Here's how the part is built. I have some questions about the finished solid (model axes, mm). A direction names the side the tool comes from. Round coordinates to 2 decimals unless told otherwise and drop trailing zeros. Loops run counter-clockwise (first coordinate to the right, second up) from the corner with the lowest first, then second, coordinate; pieces in that order, holes last. Notation, with made-up numbers: (8, 44) - (34, 44) arc R30 ccw to (34, 74) - close; hole circle Ø8 at (-24.75, -0.75). An arc over 180 degrees is marked (long way). Return JSON: item names as keys, results as strings. Group by question number.
```python
from build123d import *

# Parameters (mm, degrees)
SKETCH001_W  = 6
SKETCH001_H  = 6
PAD001_DEPTH = 0.1
FILLET001_R  = 0.3
PAD008_DEPTH = 0.7
FILLET003_R  = 0.29
PAD009_DEPTH = 0.7
FILLET004_R  = 0.29
PAD010_DEPTH = 0.7
FILLET005_R  = 0.29
SKETCH_W     = 6
SKETCH_H     = 6
PAD_DEPTH    = 3.5
FILLET_R     = 0.3
SKETCH004_R  = 0.5
PAD003_DEPTH = 0.6
SKETCH003_R  = 0.5
PAD004_DEPTH = 0.6
SKETCH005_R  = 0.5
PAD002_DEPTH = 0.6
SKETCH002_R  = 0.5
PAD005_DEPTH = 0.6
SKETCH006_R  = 1.75
PAD006_DEPTH = 0.8
FILLET006_R  = 0.1
PAD007_DEPTH = 0.7
FILLET002_R  = 0.29


with BuildPart() as fillet001:
    # Sketch001 → Pad001 (new body)
    with BuildSketch(Plane.XY.offset(3.5)):
        with Locations((3.15, -2.25)):
            Rectangle(SKETCH001_W, SKETCH001_H)
    extrude(amount=PAD001_DEPTH)

    # Fillet001
    fillet001_edges = [fillet001.edges().sort_by_distance(p)[0] for p in [
        (6.15, -5.25, 3.55),
        (0.15, -5.25, 3.55),
        (6.15, 0.75, 3.55),
        (0.15, 0.75, 3.55),
    ]]
    fillet(fillet001_edges, radius=FILLET001_R)


with BuildPart() as fillet003:
    # Sketch008 → Pad008 (new body)
    with BuildSketch(Plane.XZ.offset(0.35)):
        Polygon((-0.15, 1.5), (0.15, 1.5), (0.15, -0.5), (-0.15, -1.5), (0.15, -2.5), (0.15, -3.5), (-0.15, -3.5), (-0.15, -2.5), (-0.45, -1.5), (-0.15, -0.5), align=None)
    extrude(amount=-PAD008_DEPTH)

    # Fillet003
    fillet003_edges = [fillet003.edges().sort_by_distance(p)[0] for p in [
        (-0.15, 0, -2.5),
        (-0.15, 0, -0.5),
        (-0.45, 0, -1.5),
        (-0.15, 0, 1.5),
        (0.15, 0, -0.5),
        (-0.15, 0, -1.5),
        (0.15, 0, -2.5),
    ]]
    fillet(fillet003_edges, radius=FILLET003_R)


with BuildPart() as fillet004:
    # Sketch009 → Pad009 (new body)
    with BuildSketch(Plane.XZ.offset(4.85)):
        Polygon((6.45, 1.5), (6.15, 1.5), (6.15, -0.5), (6.45, -1.5), (6.15, -2.5), (6.15, -3.5), (6.45, -3.5), (6.45, -2.5), (6.75, -1.5), (6.45, -0.5), align=None)
    extrude(amount=-PAD009_DEPTH)

    # Fillet004
    fillet004_edges = [fillet004.edges().sort_by_distance(p)[0] for p in [
        (6.45, -4.5, -2.5),
        (6.45, -4.5, -0.5),
        (6.75, -4.5, -1.5),
        (6.45, -4.5, 1.5),
        (6.15, -4.5, -0.5),
        (6.45, -4.5, -1.5),
        (6.15, -4.5, -2.5),
    ]]
    fillet(fillet004_edges, radius=FILLET004_R)


with BuildPart() as fillet005:
    # Sketch010 → Pad010 (new body)
    with BuildSketch(Plane.XZ.offset(0.35)):
        Polygon((6.45, 1.5), (6.15, 1.5), (6.15, -0.5), (6.45, -1.5), (6.15, -2.5), (6.15, -3.5), (6.45, -3.5), (6.45, -2.5), (6.75, -1.5), (6.45, -0.5), align=None)
    extrude(amount=-PAD010_DEPTH)

    # Fillet005
    fillet005_edges = [fillet005.edges().sort_by_distance(p)[0] for p in [
        (6.45, 0, -2.5),
        (6.45, 0, -0.5),
        (6.75, 0, -1.5),
        (6.45, 0, 1.5),
        (6.15, 0, -0.5),
        (6.45, 0, -1.5),
        (6.15, 0, -2.5),
    ]]
    fillet(fillet005_edges, radius=FILLET005_R)


with BuildPart() as fillet_body:
    # Sketch → Pad (new body)
    with BuildSketch(Plane.XY):
        with Locations((3.15, -2.25)):
            Rectangle(SKETCH_W, SKETCH_H)
    extrude(amount=PAD_DEPTH)

    # Fillet
    fillet_edges = [fillet_body.edges().sort_by_distance(p)[0] for p in [
        (6.15, 0.75, 1.75),
        (6.15, -5.25, 1.75),
        (0.15, -5.25, 1.75),
        (0.15, 0.75, 1.75),
    ]]
    fillet(fillet_edges, radius=FILLET_R)


with BuildPart() as pad003:
    # Pad003 base: copy of Fillet body
    add(fillet_body.part)

    # Sketch004 → Pad003 (new body)
    with BuildSketch(Plane.XY.offset(3.5)):
        with Locations((5.15, -0.25)):
            Circle(SKETCH004_R)
    extrude(amount=PAD003_DEPTH)


with BuildPart() as pad004:
    # Pad004 base: copy of Fillet body
    add(fillet_body.part)

    # Sketch003 → Pad004 (new body)
    with BuildSketch(Plane.XY.offset(3.5)):
        with Locations((5.15, -4.25)):
            Circle(SKETCH003_R)
    extrude(amount=PAD004_DEPTH)


with BuildPart() as pad002:
    # Pad002 base: copy of Fillet body
    add(fillet_body.part)

    # Sketch005 → Pad002 (new body)
    with BuildSketch(Plane.XY.offset(3.5)):
        with Locations((1.15, -0.25)):
            Circle(SKETCH005_R)
    extrude(amount=PAD002_DEPTH)


with BuildPart() as pad005:
    # Pad005 base: copy of Fillet body
    add(fillet_body.part)

    # Sketch002 → Pad005 (new body)
    with BuildSketch(Plane.XY.offset(3.5)):
        with Locations((1.15, -4.25)):
            Circle(SKETCH002_R)
    extrude(amount=PAD005_DEPTH)


with BuildPart() as fillet006:
    # Pad006 base: copy of Fillet body
    add(fillet_body.part)

    # Sketch006 → Pad006 (new body)
    with BuildSketch(Plane.XY.offset(3.5)):
        with Locations((3.15, -2.25)):
            Circle(SKETCH006_R)
    extrude(amount=PAD006_DEPTH)

    # Fillet006
    fillet006_edges = [fillet006.edges().sort_by_distance(p)[0] for p in [
        (1.4, -2.25, 4.3),
    ]]
    fillet(fillet006_edges, radius=FILLET006_R)


with BuildPart() as obj1:
    # Sketch007 → Pad007 (new body)
    with BuildSketch(Plane.XZ.offset(4.85)):
        Polygon((-0.15, 1.5), (0.15, 1.5), (0.15, -0.5), (-0.15, -1.5), (0.15, -2.5), (0.15, -3.5), (-0.15, -3.5), (-0.15, -2.5), (-0.45, -1.5), (-0.15, -0.5), align=None)
    extrude(amount=-PAD007_DEPTH)

    # Fillet002
    fillet002_edges = [obj1.edges().sort_by_distance(p)[0] for p in [
        (-0.15, -4.5, -2.5),
        (-0.15, -4.5, -0.5),
        (-0.45, -4.5, -1.5),
        (-0.15, -4.5, 1.5),
        (0.15, -4.5, -0.5),
        (-0.15, -4.5, -1.5),
        (0.15, -4.5, -2.5),
    ]]
    fillet(fillet002_edges, radius=FILLET002_R)

    add(fillet001.part)
    add(fillet003.part)
    add(fillet004.part)
    add(fillet005.part)
    add(pad003.part)
    add(pad004.part)
    add(pad002.part)
    add(pad005.part)
    add(fillet006.part)


solid = obj1.part
```
Q1. Imagine slicing it at D-D, the plane z = -1.75. List the corners of the cut face in (x, y) for me (3 decimals), and give its area (3 significant figures).
Q2. Imagine slicing it at A-A, the plane z = 1. List the corners of the cut face in (x, y) for me.
Q3. For faces 4 (the flat face through (3, -2, 0)), 5 (the flat face through (5, -4, 4.1)), 6 (the flat face through (6.15, -2, 2)), 7 (the cylindrical face through (5.627, -0.1, 3.846)), 8 (the flat face through (0.15, -2, 2)), which set-ups out of +Z, -Z, +X, -X, +Y, -Y let a thin tool reach every point of the face, with its end or its side?
Q4. If we mould it in two halves opening along Y, with no side actions, what happens to faces 1 (the cylindrical face through (1.627, -0.1, 3.846)), 2 (the flat face through (3, -5.25, 2)), 3 (the flat face through (1, -4, 4.1))? For each: +Y half, -Y half, draft (parallel to the pull), parting line (faces both ways), or undercut.
Q5. Imagine slicing it at C-C, the plane x = 3.15. List the corners of the cut face in (y, z) for me.
Q6. Imagine slicing it at B-B, the plane y = -2.25. List the corners of the cut face in (x, z) for me, and give its area (3 significant figures).
Q7. Please list where these lines run through material, in increasing order: line 1 (X direction, y = -0.2, z = -2.75); line 2 (Z direction, x = 4, y = -2.55); line 3 (X direction, y = -3.3, z = 1).
Q8. Will these pins go through, and if not, where does the flat tip stop? pin 1 Ø0.6 at (y, z) = (-4.5, -3) entering from -X; pin 2 Ø0.6 at (y, z) = (0, 0.5) entering from +X; pin 3 Ø1.8 at (y, z) = (-1, 1.5) entering from -X; pin 4 Ø1 at (x, y) = (5, -1.5) entering from +Z.
Output values:
{
 "1": {"outline": "(-0.375, -4.85) - (-0.075, -4.85) - (-0.075, -4.15) - (-0.375, -4.15) - close; (-0.375, -0.35) - (-0.075, -0.35) - (-0.075, 0.35) - (-0.375, 0.35) - close; (6.375, -4.85) - (6.675, -4.85) - (6.675, -4.15) - (6.375, -4.15) - close; (6.375, -0.35) - (6.675, -0.35) - (6.675, 0.35) - (6.375, 0.35) - close", "area": "0.840 mm^2"},
 "2": {"outline": "(-0.15, -4.85) - (0.15, -4.85) - (0.15, -4.95) arc R0.3 ccw to (0.45, -5.25) - (5.85, -5.25) arc R0.3 ccw to (6.15, -4.95) - (6.15, -4.85) - (6.45, -4.85) - (6.45, -4.15) - (6.15, -4.15) - (6.15, -0.35) - (6.45, -0.35) - (6.45, 0.35) - (6.15, 0.35) - (6.15, 0.45) arc R0.3 ccw to (5.85, 0.75) - (0.45, 0.75) arc R0.3 ccw to (0.15, 0.45) - (0.15, 0.35) - (-0.15, 0.35) - (-0.15, -0.35) - (0.15, -0.35) - (0.15, -4.15) - (-0.15, -4.15) - close"},
 "3": {"face 4": "-Z, +Y, -Y", "face 5": "+Z, +X, -Y", "face 6": "+Z, +X", "face 7": "+Z", "face 8": "+Z, -X"},
 "4": {"face 1": "undercut", "face 2": "-Y half", "face 3": "draft"},
 "5": {"outline": "(-5.25, 0) - (0.75, 0) - (0.75, 3.6) - (-0.5, 3.6) - (-0.5, 4.2) arc R0.1 ccw to (-0.6, 4.3) - (-3.9, 4.3) arc R0.1 ccw to (-4, 4.2) - (-4, 3.6) - (-5.25, 3.6) - close"},
 "6": {"outline": "(0.15, 0) - (6.15, 0) - (6.15, 3.6) - (4.9, 3.6) - (4.9, 4.2) arc R0.1 ccw to (4.8, 4.3) - (1.5, 4.3) arc R0.1 ccw to (1.4, 4.2) - (1.4, 3.6) - (0.15, 3.6) - close", "area": "24.0 mm^2"},
 "7": {"line 1": "x = -0.15 to 0.15, 6.15 to 6.45", "line 2": "z = 0 to 4.3", "line 3": "x = 0.15 to 6.15"},
 "8": {"pin 1": "stops at x = -0.15", "pin 2": "stops at x = 6.45", "pin 3": "stops at x = -0.15", "pin 4": "stops at z = 4.3"}
}
